Autodesk Inventor part; units mm, degrees
ref_plane "YZ Plane" through (0, 0, 0) normal (1, 0, 0) x (0, 1, 0)
ref_plane "XZ Plane" through (0, 0, 0) normal (0, 1, 0) x (-1, 0, 0)
ref_plane "XY Plane" through (0, 0, 0) normal (0, 0, 1) x (1, 0, 0)
sketch "Sketch1" plane through (0, 0, 0) normal (0, 1, 0) x (-1, 0, 0)
  line L0 (-20, -20) -> (20, -20)
  line L1 (20, -20) -> (20, 20)
  line L2 (20, 20) -> (-20, 20)
  line L3 (-20, 20) -> (-20, -20)
  line L4 (-20, -20) -> (20, 20) construction
  line L5 (20, -20) -> (-20, 20) construction
  point P0 (0, 0)
  dimension "d0" = 40
  dimension "d1" = 40
extrude "Plate1" add sketch "Sketch1" along normal blind 0.5
sketch "Sketch2" plane through (20, 0, 19.5) normal (0, 0, 1) x (1, 0, 0)
  line L0 (-40, 0) -> (0, 0)
  line L1 (0, 0) -> (0, 50)
  line L2 (0, 50) -> (-40, 50)
  line L3 (-40, 50) -> (-40, 0)
edge flange "Flange1" height 50 angle 90 thickness 0.5 bend radius 0.5 thickness toward (0, 0, 1) relief tear relief width 0.5 relief depth 0.25 edges at (0, 0.5, 20) wall of the first edge with corners at (-20, 0, 19.5) (20, 0, 19.5) (20, 50, 19.5) (-20, 50, 19.5)
bend "Bend1"
corner "Corner1"
sketch "Sketch3" plane through (20, 50, 19.5) normal (0, 0, -1) x (-1, 0, 0)
  line L0 (40, 0) -> (0, 0) construction
  line L1 (20, 0) -> (20, -49) construction
  line L2 (0, -49) -> (40, -49) construction
  line L3 (0, 0) -> (0, -20) construction
  line L4 (0, 0) -> (0, -49) construction
  line L5 (0, -20) -> (0, -40) construction
  line L6 (40, 0) -> (40, -49) construction
  line L7 (0, 0) -> (1.6205, 0)
  line L8 (0, 0) -> (0, -15) construction
  line L9 (0, -15) -> (20, -15) construction
  circle A0 centre (20, -15) radius 5 construction
  line L10 (0, -15) -> (0, -35) construction
  line L11 (0, -35) -> (20, -35) construction
  circle A1 centre (20, -35) radius 5 construction
  point P0 (20, -50)
  dimension "d15" = 15
  dimension "d16" = 20
hole "Hole1" at (0, 35, 19.5) at (0, 15, 19.5) direction (0, 0, 1) diameter 10 end through all
sketch "Sketch4" plane through (0, 0.5, 0) normal (0, 1, 0) x (1, 0, 0)
  point P0 (0, 0)
hole "Hole2" at (0, 0.5, 0) direction (0, -1, 0) diameter 9.254 end through all
equation "\"d22\" = Thickness"
equation "\"d29\" = Thickness"
equation "\"d3\" = BendReliefWidth"
equation "\"d4\" = BendReliefDepth"
equation "\"d5\" = MinimumRemnant"
equation "\"d6\" = BendRadius"
equation "\"d9\" = BendRadius"
equation "\"d10\" = CornerReliefSize"
equation "\"d11\" = GapSize"
equation "\"d12\" = JacobiRadiusSize"
equation "\"BendRadius\" = Thickness"
equation "\"BendReliefWidth\" = Thickness"
equation "\"BendReliefDepth\" = 0.5 * Thickness"
equation "\"CornerReliefSize\" = 4 * Thickness"
equation "\"MinimumRemnant\" = 2 * Thickness"
equation "\"TransitionRadius\" = BendRadius"
equation "\"JacobiRadiusSize\" = BendRadius"
equation "\"GapSize\" = Thickness"
equation "\"d2\" = BendRadius"
properties part number "L Braket for Wheels"
Check sheet for the modelled part. Datum: model origin and axes. Units: mm. A direction names the side the tool comes from. Give positions to 0.01 mm unless a question says otherwise; leave off trailing zeros. Order: outer loops, then holes, each group sorted by start corner. A loop starts at its lowest first (then second) coordinate and runs counter-clockwise, first axis right, second up. Notation, with made-up numbers: M -10.5,44.5 L 20.5,44.5 A23 ccw 20.5,79.5 Z; hole C -10,-22.5 d2. An arc over 180 degrees is marked long. Answer in a Markdown table with one row per item.
1) Cross-section at A-A, the plane z = 0. Enter the section's corners in (x, y).
Filled sheet:
| item | result |
|---|---|
| outline | M -20,0 L -4.63,0 L -4.63,0.5 L -20,0.5 Z; M 4.63,0 L 20,0 L 20,0.5 L 4.63,0.5 Z |
2) Cross-section at D-D, the plane x = -10. Enter the section's corners in (y, z), plus the area to 3 significant figures.
Filled sheet:
| item | result |
|---|---|
| outline | M 0,-20 L 0.5,-20 L 0.5,19 A0.5 cw 1,19.5 L 50,19.5 L 50,20 L 1,20 A1 ccw 0,19 Z |
| area | 44.6 mm2 |
3) Gauge pin test, flat ends, axial feed: P1, Ø12, axis at x = -9.5, z = 6.5, coming from the +Y side; P2, Ø16, axis at x = 0, y = 15, coming from the +Z side; P3, Ø1.5, axis at x = -15, y = 20.5, coming from the -Z side. Record the tip position at first contact, or that the pin passes through.
Filled sheet:
| item | result |
|---|---|
| P1 | stops at y = 0.5 |
| P2 | stops at z = 20 |
| P3 | stops at z = 19.5 |
4) Cross-section at B-B, the plane x = 0. Enter the section's corners in (y, z), plus the area to 3 significant figures.
Filled sheet:
| item | result |
|---|---|
| outline | M 0,-20 L 0.5,-20 L 0.5,-4.63 L 0,-4.63 Z; M 0,4.63 L 0.5,4.63 L 0.5,19 A0.5 cw 1,19.5 L 10,19.5 L 10,20 L 1,20 A1 ccw 0,19 Z; M 20,19.5 L 30,19.5 L 30,20 L 20,20 Z; M 40,19.5 L 50,19.5 L 50,20 L 40,20 Z |
| area | 30.0 mm2 |
5) Cross-section at C-C, the plane y = 35. Enter the section's corners in (x, z), plus the area to 3 significant figures.
Filled sheet:
| item | result |
|---|---|
| outline | M -20,19.5 L -5,19.5 L -5,20 L -20,20 Z; M 5,19.5 L 20,19.5 L 20,20 L 5,20 Z |
| area | 15.0 mm2 |
6) Release check for a two-part mould opening along Y. For faces 3 (the flat face through (5, 0.5, 0)), 4 (the cylindrical face through (-0.22, 30.005, 19.754)), 5 (the cylindrical face through (4.517, 0.246, -1.003)) record: +Y half, -Y half, draft (parallel to the pull), parting line (faces both ways), or undercut.
Filled sheet:
| item | result |
|---|---|
| face 3 | +Y half |
| face 4 | undercut |
| face 5 | draft |
7) Thickness scan on L1, parallel to Y at x = 0, z = 19.9; L2, parallel to Y at x = 0, z = 19; L3, parallel to X at y = 0.1, z = 0. Record the ranges inside material, lowest first. Write a range as [from, to].
Filled sheet:
| item | result |
|---|---|
| L1 | y = [0.56, 10], [20, 30], [40, 50] |
| L2 | y = [0, 0.5] |
| L3 | x = [-20, -4.63], [4.63, 20] |
8) Access from +Z, -Z, +X, -X, +Y, -Y to the whole of each face (thin tool, end or side, straight path). Record for faces 1 (the flat face through (0, 25, 19.5)), 2 (the flat face through (0, 26, 20)).
Filled sheet:
| item | result |
|---|---|
| face 1 | -Z, +X, -X, +Y |
| face 2 | +Z, +X, -X, +Y, -Y |
